from build123d import *

# Parameters (mm, degrees)
SKETCH1_W                                         = 53.975
SKETCH1_H                                         = 53.975
SKETCH1_W_2                                       = 50.8
SKETCH1_H_2                                       = 50.8
BOSS_EXTRUDE1_DEPTH                               = 6.35
SKETCH2_W                                         = 53.975
SKETCH2_H                                         = 53.975
BOSS_EXTRUDE2_DEPTH                               = 2.38125
BOSS_EXTRUDE3_DEPTH                               = 3.2512
BOSS_EXTRUDE3_DEPTH_BACK                          = 1.5875
CSK_FOR_8_FLAT_HEAD_MACHINE_SCREW_100_D           = 4.4958
CSK_FOR_8_FLAT_HEAD_MACHINE_SCREW_100_CSINK_D     = 8.4328
CSK_FOR_8_FLAT_HEAD_MACHINE_SCREW_100_CSINK_ANGLE = 100
SKETCH7_W                                         = 41.148
SKETCH7_H                                         = 41.148
CUT_EXTRUDE1_DEPTH                                = 7.35
CUT_EXTRUDE1_DEPTH_BACK                           = 6.63245
FILLET2_R                                         = 9.525
BOSS_EXTRUDE4_DEPTH                               = 7.14375
CUT_EXTRUDE2_DEPTH                                = 12.98245
FILLET3_R                                         = 0.79375


with BuildPart() as part:
    # Sketch1 → Boss-Extrude1 (new body)
    with BuildSketch(Plane(origin=(0, 0, 0), x_dir=(1, 0, 0), z_dir=(0, 1, 0))):
        Rectangle(SKETCH1_W, SKETCH1_H)
        Rectangle(SKETCH1_W_2, SKETCH1_H_2, mode=Mode.SUBTRACT)
    extrude(amount=BOSS_EXTRUDE1_DEPTH)

    # Sketch2 → Boss-Extrude2 (add)
    with BuildSketch(Plane.XZ):
        Rectangle(SKETCH2_W, SKETCH2_H)
    extrude(amount=BOSS_EXTRUDE2_DEPTH)

    # Sketch3 → Boss-Extrude3 (add, two sides)
    with BuildSketch(Plane.XZ.offset(2.38125)) as boss_extrude3_sk:
        Polygon((-26.9875, 26.590625), (26.590625, 26.590625), (26.590625, -26.9875), (28.178125, -26.9875), (28.178125, 28.178125), (-26.9875, 28.178125), align=None)
    extrude(amount=BOSS_EXTRUDE3_DEPTH)
    extrude(boss_extrude3_sk.sketch, amount=-BOSS_EXTRUDE3_DEPTH_BACK)

    # CSK for #8 Flat Head Machine Screw (100)1 (through all)
    with Locations(Plane(origin=(19.05, 0, 19.05), x_dir=(0, 0, 1), z_dir=(0, 1, 0))):
        with Locations((0, 0), (-38.1, -38.1), (-38.1, 0), (0, -38.1)):
            CounterSinkHole(CSK_FOR_8_FLAT_HEAD_MACHINE_SCREW_100_D / 2, CSK_FOR_8_FLAT_HEAD_MACHINE_SCREW_100_CSINK_D / 2, counter_sink_angle=CSK_FOR_8_FLAT_HEAD_MACHINE_SCREW_100_CSINK_ANGLE)

    # Sketch7 → Cut-Extrude1 (cut, two sides)
    with BuildSketch(Plane(origin=(0, 0, 0), x_dir=(1, 0, 0), z_dir=(0, 1, 0))) as cut_extrude1_sk:
        with Locations((-6.4135, 6.4135)):
            Rectangle(SKETCH7_W, SKETCH7_H)
    extrude(amount=CUT_EXTRUDE1_DEPTH, mode=Mode.SUBTRACT)
    extrude(cut_extrude1_sk.sketch, amount=-CUT_EXTRUDE1_DEPTH_BACK, mode=Mode.SUBTRACT)

    # Fillet2
    fillet2_edges = [part.edges().sort_by_distance(p)[0] for p in [
        (14.1605, -1.190625, 14.1605),
    ]]
    fillet(fillet2_edges, radius=FILLET2_R)

    # Sketch8 → Boss-Extrude4 (add)
    with BuildSketch(Plane(origin=(0, -0.79375, 0), x_dir=(1, 0, 0), z_dir=(0, 1, 0))):
        Polygon((28.178125, 26.9875), (26.9875, 26.9875), (26.9875, -26.9875), (-26.9875, -26.9875), (-26.9875, -28.178125), (28.178125, -28.178125), align=None)
    extrude(amount=BOSS_EXTRUDE4_DEPTH)

    # Sketch9 → Cut-Extrude2 (cut, through all)
    with BuildSketch(Plane.XZ.offset(5.63245)):
        Polygon((-26.9875, 28.178125), (-26.9875, 26.590625), (26.590625, 26.590625), (26.590625, -26.9875), (28.178125, -26.9875), (28.178125, 28.178125), align=None)
    extrude(amount=-CUT_EXTRUDE2_DEPTH, mode=Mode.SUBTRACT)

    # Fillet3
    fillet3_edges = [part.edges().sort_by_distance(p)[0] for p in [
        (26.590625, 1.984375, -26.9875),
        (26.590625, 1.984375, 26.590625),
        (-26.9875, 1.984375, 26.590625),
        (25.4, 0, 0),
        (25.4, 3.175, 25.4),
        (19.78025, 0, -25.4),
        (25.4, 3.175, -25.4),
        (0, 0, 25.4),
        (-25.4, 3.175, 25.4),
        (-25.4, 0, 19.78025),
    ]]
    fillet(fillet3_edges, radius=FILLET3_R)


solid = part.part
CAD build for the part. Positions are in the model's coordinates, mm. A direction names the side the tool comes from. Give positions to 0.01 mm unless a question says otherwise; leave off trailing zeros. Loops run counter-clockwise (first coordinate to the right, second up) from the corner with the lowest first, then second, coordinate; pieces in that order, holes last. Notation, with made-up numbers: M 71.25,74.25 L 94.25,74.25 A22 cw 94.25,101.25 Z; hole C 52,-5 d11. An arc over 180 degrees is marked long. One line per question, with ' | ' between items. Start each with the question number.
1. Saw through at B-B on z = -19.05. Give the cut face in (x, y), plus the area to 3 significant figures.
2. Flat gauge pins, fed straight in: pin 1 (4.5 mm diameter, centred on y = 5, z = 8, fed in from -X); pin 2 (1.5 mm diameter, centred on x = 11, y = -0.5, fed in from -Z); pin 3 (3 mm diameter, centred on x = 4, y = 2.5, fed in from -Z). Where does each tip first touch, or does it go through?
3. Probe L1, parallel to Z at x = 19.05, y = -2.2; L2, parallel to X at y = 1, z = 19. List the from-to ranges inside material, lowest first. Write a range as from..to.
4. Saw through at D-D on x = 19.05. Give the cut face in (y, z), plus the area to 3 significant figures.
5. 3-axis set-ups, long thin cutter, end or side, ignore diameter. For faces 1 (the face through (-25.4, 4, 19)), 2 (the face through (13, 0, 13)), 3 (the face through (-15, -1, 14.161)): which of +Z, -Z, +X, -X, +Y, -Y reach the whole face in a straight line?
6. Saw through at C-C on z = 19.05. Give the cut face in (x, y), plus the area to 3 significant figures.
7. Two-plate mould, pull along Z, no slides. Class faces 4 (the face through (-26.988, 2, 20)), 5 (the face through (19.7, -2, 16.9)), 6 (the face through (11.44, -1.21, 11.3)): pulls with the +Z half, pulls with the -Z half, needs draft (parallel to the pull), parting line crosses it, or undercut.
8. Saw through at A-A on x = -19.05. Give the cut face in (y, z), plus the area to 3 significant figures.
Result sheet:
1) outline: M 14.16,-2.38 L 16.8,-2.38 L 16.8,-1.65 L 14.83,0 L 14.16,0 Z; M 21.3,-2.38 L 26.59,-2.38 L 26.59,6.35 L 25.4,6.35 L 25.4,0.79 A0.79 cw 24.61,0 L 23.27,0 L 21.3,-1.65 Z | area: 23.3 mm^2
2) pin 1: stops at x = 25.4 | pin 2: stops at z = 10.97 | pin 3: stops at z = 25.4
3) L1: z = -26.99..-21.3, -16.8..16.8, 21.3..26.59 | L2: x = -26.99..-25.4, 25.4..26.59
4) outline: M -2.38,-26.99 L 6.35,-26.99 L 6.35,-25.4 L 0.79,-25.4 A0.79 cw 0,-24.61 L 0,-23.27 L -1.65,-21.3 L -2.38,-21.3 Z; M -2.38,-16.8 L -1.65,-16.8 L 0,-14.83 L 0,14.83 L -1.65,16.8 L -2.38,16.8 Z; M -2.38,21.3 L -1.65,21.3 L 0,23.27 L 0,24.61 A0.79 cw 0.79,25.4 L 6.35,25.4 L 6.35,26.59 L -2.38,26.59 Z | area: 118 mm^2
5) face 1: -Z, +Y | face 2: +Y | face 3: -Z, -X, +Y, -Y
6) outline: M -26.99,-2.38 L -21.3,-2.38 L -21.3,-1.65 L -23.27,0 L -24.61,0 A0.79 cw -25.4,0.79 L -25.4,6.35 L -26.99,6.35 Z; M -16.8,-2.38 L 16.8,-2.38 L 16.8,-1.65 L 14.83,0 L -14.83,0 L -16.8,-1.65 Z; M 21.3,-2.38 L 26.59,-2.38 L 26.59,6.35 L 25.4,6.35 L 25.4,0.79 A0.79 cw 24.61,0 L 23.27,0 L 21.3,-1.65 Z | area: 118 mm^2
7) face 4: needs draft | face 5: undercut | face 6: pulls with the -Z half
8) outline: M -2.38,14.16 L 0,14.16 L 0,14.83 L -1.65,16.8 L -2.38,16.8 Z; M -2.38,21.3 L -1.65,21.3 L 0,23.27 L 0,24.61 A0.79 cw 0.79,25.4 L 6.35,25.4 L 6.35,26.59 L -2.38,26.59 Z | area: 23.3 mm^2
